For this review, take the finished solid that the model builds, in its own axes (mm). Round coordinates to 2 decimals unless told otherwise and drop trailing zeros. Order: outer loops, then holes, each group sorted by start corner. A loop starts at its lowest first (then second) coordinate and runs counter-clockwise, first axis right, second up. Notation, with made-up numbers: (4, 18.25) - (34, 18.25) arc R12 ccw to (34, 26.25) - close; hole circle Ø7 at (72.25, 37). An arc over 180 degrees is marked (long way). Write each question's results on one line, items separated by ' | '. Start each with the question number.
(1) Take a section at B-B, the plane x = -13. Give the boundary of the cut face in (y, z) (3 decimals), plus the area to 3 significant figures.
(2) Take a section at A-A, the plane x = 7.62. Give the boundary of the cut face in (y, z) (3 decimals).
(3) For L1, parallel to X at y = 4, z = -1.75; L2, parallel to X at y = 1, z = -0.35; L3, parallel to X at y = 0.75, z = -1.5, list the stretches that pass through material, from the lowest coordinate up. Write a range as from..to.
(4) Insertion check: pin 1 Ø0.6 at (x, z) = (-5.5, -2) entering from +Y. The pin has a flat end and moves straight along its axis. Give the tip position at first contact, or say it passes through.
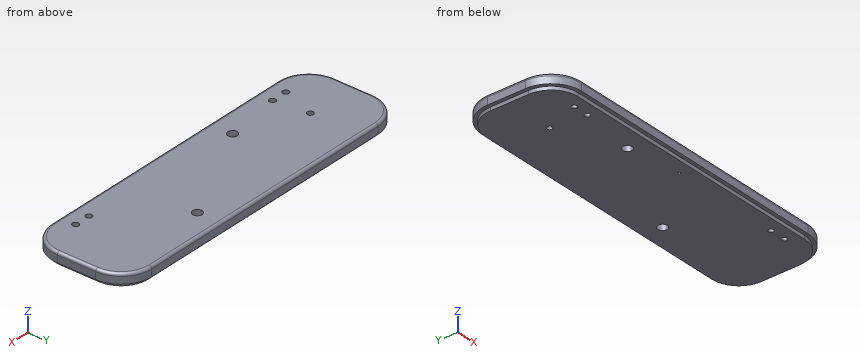
```python
from build123d import *

# Parameters (mm, degrees)
SKETCH1_W           = 47.6504
SKETCH1_H           = 14.224
BOSS_EXTRUDE1_DEPTH = 1.397
SKETCH2_W           = 46.6344
SKETCH2_H           = 13.208
BOSS_EXTRUDE2_DEPTH = 0.508
FILLET1_R           = 3.8608
FILLET2_R           = 3.8608
FILLET3_R           = 3.8608
FILLET4_R           = 3.8608
FILLET5_R           = 4.3688
FILLET6_R           = 4.3688
FILLET7_R           = 4.3688
FILLET8_R           = 4.3688
FILLET9_R           = 0.381
LPATTERN1_COUNT     = 2
LPATTERN1_PITCH     = 2.286
SKETCH7_R           = 0.6731
CUT_EXTRUDE1_DEPTH  = 25.936914886
SKETCH8_R           = 0.17145
CUT_EXTRUDE2_DEPTH  = 1.27


with BuildPart() as part:
    # Sketch1 → Boss-Extrude1 (new body)
    with BuildSketch(Plane(origin=(0, 0, -1.397), x_dir=(-1, 0, 0), z_dir=(0, 0, -1))):
        Rectangle(SKETCH1_W, SKETCH1_H)
    extrude(amount=-BOSS_EXTRUDE1_DEPTH)

    # Sketch2 → Boss-Extrude2 (add)
    with BuildSketch(Plane(origin=(0, 0, -1.397), x_dir=(-1, 0, 0), z_dir=(0, 0, -1))):
        Rectangle(SKETCH2_W, SKETCH2_H)
    extrude(amount=BOSS_EXTRUDE2_DEPTH)

    # Sketch3 → Cut-Revolve1 (revolve, cut)
    with BuildSketch(Plane.XZ, mode=Mode.PRIVATE) as cut_revolve1_sk:
        Polygon((-15.9512, 0), (-16.3957, 0), (-16.3957, -1.905), (-16.0147, -1.905), (-16.0147, -1.651), (-15.9512, -1.651), align=None)
    revolve(cut_revolve1_sk.sketch.rotate(Axis((-16.3957, 0, 0), (0, 0, -1)), 180), axis=Axis((-16.3957, 0, 0), (0, 0, -1)), mode=Mode.SUBTRACT)

    # Sketch6 → Cut-Revolve4 (revolve, cut)
    with BuildSketch(Plane.XZ.offset(4.9022), mode=Mode.PRIVATE) as cut_revolve4_sk:
        Polygon((-15.3543, 0), (-15.7988, 0), (-15.7988, -1.905), (-15.4178, -1.905), (-15.4178, -1.778), (-15.3543, -1.778), align=None)
    cut_revolve4 = revolve(cut_revolve4_sk.sketch.rotate(Axis((-15.7988, -4.9022, 0), (0, 0, -1)), 180), axis=Axis((-15.7988, -4.9022, 0), (0, 0, -1)), mode=Mode.SUBTRACT)

    # Fillet1
    fillet1_edges = [part.edges().sort_by_distance(p)[0] for p in [
        (23.3172, -6.604, -1.651),
    ]]
    fillet(fillet1_edges, radius=FILLET1_R)

    # Fillet2
    fillet2_edges = [part.edges().sort_by_distance(p)[0] for p in [
        (-23.3172, -6.604, -1.651),
    ]]
    fillet(fillet2_edges, radius=FILLET2_R)

    # Fillet3
    fillet3_edges = [part.edges().sort_by_distance(p)[0] for p in [
        (-23.3172, 6.604, -1.651),
    ]]
    fillet(fillet3_edges, radius=FILLET3_R)

    # Fillet4
    fillet4_edges = [part.edges().sort_by_distance(p)[0] for p in [
        (23.3172, 6.604, -1.651),
    ]]
    fillet(fillet4_edges, radius=FILLET4_R)

    # Fillet5
    fillet5_edges = [part.edges().sort_by_distance(p)[0] for p in [
        (-23.8252, -7.112, -0.6985),
    ]]
    fillet(fillet5_edges, radius=FILLET5_R)

    # Fillet6
    fillet6_edges = [part.edges().sort_by_distance(p)[0] for p in [
        (-23.8252, 7.112, -0.6985),
    ]]
    fillet(fillet6_edges, radius=FILLET6_R)

    # Fillet7
    fillet7_edges = [part.edges().sort_by_distance(p)[0] for p in [
        (23.8252, 7.112, -0.6985),
    ]]
    fillet(fillet7_edges, radius=FILLET7_R)

    # Fillet8
    fillet8_edges = [part.edges().sort_by_distance(p)[0] for p in [
        (23.8252, -7.112, -0.6985),
    ]]
    fillet(fillet8_edges, radius=FILLET8_R)

    # Fillet9
    fillet9_edges = [part.edges().sort_by_distance(p)[0] for p in [
        (-23.8252, 0, 0),
        (-22.545608106, -5.832408106, 0),
        (0, 7.112, 0),
        (-22.545608106, 5.832408106, 0),
        (23.8252, 0, 0),
        (22.545608106, 5.832408106, 0),
        (0, -7.112, 0),
        (22.545608106, -5.832408106, 0),
    ]]
    fillet(fillet9_edges, radius=FILLET9_R)

    # LPattern1: Cut-Revolve4 ×2
    with Locations(*[(-i * LPATTERN1_PITCH, 0, 0) for i in range(1, LPATTERN1_COUNT)]):
        add(cut_revolve4, mode=Mode.SUBTRACT)

    # Mirror1: Cut-Revolve4 across plane
    add(cut_revolve4.mirror(Plane(origin=(0, 0, 0), x_dir=(0, 0, 1), z_dir=(1, 0, 0))), mode=Mode.SUBTRACT)

    # Mirror1 copy 1 sketch → Mirror1 copy 1 (revolve, cut)
    with BuildSketch(Plane(origin=(2.286, -4.9022, 0), x_dir=(-1, 0, 0), z_dir=(0, -1, 0))):
        Polygon((-15.3543, 0), (-15.7988, 0), (-15.7988, 1.905), (-15.4178, 1.905), (-15.4178, 1.778), (-15.3543, 1.778), align=None)
    revolve(axis=Axis((18.0848, -4.9022, 0), (0, 0, 1)), mode=Mode.SUBTRACT)

    # Sketch7 → Cut-Extrude1 (cut, through all)
    with BuildSketch(Plane.XY):
        with Locations((-7.62, -3.81)):
            Circle(SKETCH7_R)
        with Locations((7.62, 3.81)):
            Circle(SKETCH7_R)
    extrude(amount=-CUT_EXTRUDE1_DEPTH, mode=Mode.SUBTRACT)

    # Sketch8 → Cut-Extrude2 (cut)
    with BuildSketch(Plane(origin=(0, 0, -1.905), x_dir=(-1, 0, 0), z_dir=(0, 0, -1))):
        with Locations((0, -4.9022)):
            Circle(SKETCH8_R)
    extrude(amount=-CUT_EXTRUDE2_DEPTH, mode=Mode.SUBTRACT)


solid = part.part
```
Results below:
1) outline: (-7.112, -1.397) - (-6.604, -1.397) - (-6.604, -1.905) - (6.604, -1.905) - (6.604, -1.397) - (7.112, -1.397) - (7.112, -0.381) arc R0.381 ccw to (6.731, 0) - (-6.731, 0) arc R0.381 ccw to (-7.112, -0.381) - close | area: 26.5 mm^2
2) outline: (-7.112, -1.397) - (-6.604, -1.397) - (-6.604, -1.905) - (3.137, -1.905) - (3.137, 0) - (-6.731, 0) arc R0.381 ccw to (-7.112, -0.381) - close; (4.483, -1.905) - (6.604, -1.905) - (6.604, -1.397) - (7.112, -1.397) - (7.112, -0.381) arc R0.381 ccw to (6.731, 0) - (4.483, 0) - close
3) L1: x = -23.11..6.97, 8.27..23.11 | L2: x = -23.82..23.82 | L3: x = -23.32..23.32
4) pin 1: stops at y = 6.6
